from build123d import *

# Parameters (mm, degrees)
F0_W     = 1066.8
F0_H     = 342.9
F1_DEPTH = 50.8
F3_DEPTH = 50.8
F4_R     = 38.1
F6_DEPTH = 50.8
F8_DEPTH = 50.8


with BuildPart() as f1:
    # F0 (on Top) → F1 (new body)
    with BuildSketch(Plane.XY):
        Rectangle(F0_W, F0_H)
    extrude(amount=F1_DEPTH)

    # F2 (on face) → F3 (cut)
    with BuildSketch(Plane.XY.offset(50.8)):
        Polygon((-317.5, -114.3), (-317.5, -171.45), (-285.75, -171.45), (-285.75, -101.6), (-28.575, -101.6), (-28.575, -44.45), (412.75, -44.45), (412.75, 82.55), (-28.575, 82.55), (-28.575, 139.7), (-365.125, 139.7), (-403.225, 101.537321), (-403.225, 31.75), (-501.65, 31.75), (-501.65, 0), (-403.225, 0), (-403.225, -114.3), align=None)
    extrude(amount=-F3_DEPTH, mode=Mode.SUBTRACT)

    # F4
    f4_edges = [f1.edges().sort_by_distance(p)[0] for p in [
        (-533.4, 171.45, 25.4),
        (-533.4, -171.45, 25.4),
        (533.4, 171.45, 25.4),
        (533.4, -171.45, 25.4),
    ]]
    fillet(f4_edges, radius=F4_R)

    # F5 (on face) → F6 (cut)
    with BuildSketch(Plane.XY.offset(50.8)):
        with BuildLine():
            Line((172.965391, -95.25), (82.55, -95.25))
            Line((82.55, -95.25), (82.55, -120.65))
            Line((82.55, -120.65), (172.965391, -120.65))
            ThreePointArc((172.965391, -120.65), (171.45, -107.95), (172.965391, -95.25))
        make_face()
        with BuildLine():
            ThreePointArc((279.4, -107.95), (231.820045, -54.355187), (172.965391, -95.25))
            ThreePointArc((172.965391, -95.25), (171.45, -107.95), (172.965391, -120.65))
            ThreePointArc((172.965391, -120.65), (231.820045, -161.544813), (279.4, -107.95))
        make_face()
    extrude(amount=-F6_DEPTH, mode=Mode.SUBTRACT)

    # F7 (on face) → F8 (cut)
    with BuildSketch(Plane.XY.offset(50.8)):
        with BuildLine():
            Line((395.215391, -95.25), (304.8, -95.25))
            Line((304.8, -95.25), (304.8, -120.65))
            Line((304.8, -120.65), (395.215391, -120.65))
            ThreePointArc((395.215391, -120.65), (393.7, -107.95), (395.215391, -95.25))
        make_face()
        with BuildLine():
            ThreePointArc((501.65, -107.95), (454.070045, -54.355187), (395.215391, -95.25))
            ThreePointArc((395.215391, -95.25), (393.7, -107.95), (395.215391, -120.65))
            ThreePointArc((395.215391, -120.65), (454.070045, -161.544813), (501.65, -107.95))
        make_face()
    extrude(amount=-F8_DEPTH, mode=Mode.SUBTRACT)


solid = f1.part
Check sheet for the modelled part. Datum: model origin and axes. Units: mm. A direction names the side the tool comes from. Round coordinates to 2 decimals unless told otherwise and drop trailing zeros. Order: outer loops, then holes, each group sorted by start corner. A loop starts at its lowest first (then second) coordinate and runs counter-clockwise, first axis right, second up.
(1) Scan lines: probe 1 along Y at (x, z) = (124, 22); probe 2 along X at (y, z) = (37.5, 35) (3 decimals); probe 3 along Y at (x, z) = (62, 33.5). Record each from-to range of solid material in increasing order.
(2) Cross-section at D-D, the plane z = 8. State how many separate pieces and enclosed holes the cut face has, and give its area (3 significant figures).
(3) Cross-section at B-B, the plane y = -63. Enter the section's corners in (x, z) (3 decimals).
(4) Cross-section at A-A, the plane x = 290.5. Enter the section's corners in (y, z).
(5) Cross-section at C-C, the plane x = -274. Enter the section's corners in (y, z), and give its area (3 significant figures).
(6) Access from +Z, -Z, +X, -X, +Y, -Y to the whole of each face (thin tool, end or side, straight path). Record for faces 4 (the flat face through (-7, 171.45, 25)), 5 (the flat face through (-452, 31.75, 26)), 6 (the flat face through (-285.75, -137, 26)).
(7) Draft check along Y on faces 1 (the cylindrical face through (-522.54, 159.99, 25.76)), 2 (the flat face through (533.4, -2, 25)), 3 (the flat face through (189, -44.45, 26)). Enter one of: pulls with the +Y half, pulls with the -Y half, needs draft (parallel to the pull), parting line crosses it, or undercut.
(8) Go/stop test with flat-tipped pins: P1, Ø15, axis at y = -147, z = 16, coming from the +X side; P2, Ø12, axis at x = -37.5, y = 81.5, coming from the +Z side. Record where each tip stops, or that it passes through.
Check sheet entries:
1. probe 1: y = -171.45 to -120.65, -95.25 to -44.45, 82.55 to 171.45
1. probe 2: x = -533.4 to -403.225, 412.75 to 533.4
1. probe 3: y = -171.45 to -44.45, 82.55 to 171.45
2. separate pieces: 1
2. enclosed holes: 2
2. area: 190,000 mm2
3. outline: (-533.4, 0) - (-403.225, 0) - (-403.225, 50.8) - (-533.4, 50.8) - close; (-28.575, 0) - (195.545, 0) - (195.545, 50.8) - (-28.575, 50.8) - close; (255.305, 0) - (417.795, 0) - (417.795, 50.8) - (255.305, 50.8) - close; (477.555, 0) - (533.4, 0) - (533.4, 50.8) - (477.555, 50.8) - close
4. outline: (-171.45, 0) - (-44.45, 0) - (-44.45, 50.8) - (-171.45, 50.8) - close; (82.55, 0) - (171.45, 0) - (171.45, 50.8) - (82.55, 50.8) - close
5. outline: (-171.45, 0) - (-101.6, 0) - (-101.6, 50.8) - (-171.45, 50.8) - close; (139.7, 0) - (171.45, 0) - (171.45, 50.8) - (139.7, 50.8) - close
5. area: 5,160 mm2
6. face 4: +Z, -Z, +X, -X, +Y
6. face 5: +Z, -Z
6. face 6: +Z, -Z, -Y
7. face 1: pulls with the +Y half
7. face 2: needs draft
7. face 3: undercut
8. P1: stops at x = 532.9
8. P2: passes through
